from build123d import *

# Parameters (mm, degrees)
F0_W     = 368.677914
F0_H     = 204.665296
F1_DEPTH = 12.7
F2_W     = 368.677914
F2_H     = 204.665296
F2_R     = 96.2279
F3_DEPTH = 12.7
F4_DEPTH = 7.62


with BuildPart() as f1:
    # F0 (on Front) → F1 (new body)
    with BuildSketch(Plane.XZ):
        with Locations((0.233635, 0.70091)):
            Rectangle(F0_W, F0_H)
    extrude(amount=F1_DEPTH)

    # F2 (on face) → F3 (cut)
    with BuildSketch(Plane.XZ.offset(12.7)):
        with Locations((0.233635, 0.70091)):
            Rectangle(F2_W, F2_H)
        Circle(F2_R, mode=Mode.SUBTRACT)
    extrude(amount=-F3_DEPTH, mode=Mode.SUBTRACT)

    # F2 (on face) + F0 (on Front) → F4 (cut)
    with BuildSketch(Plane.XZ.offset(12.7)):
        Circle(F2_R)
    with BuildSketch(Plane.XZ):
        with Locations((0.233635, 0.70091)):
            Rectangle(F0_W, F0_H)
    extrude(amount=-F4_DEPTH, mode=Mode.SUBTRACT)


solid = f1.part
The listing builds one solid part. Answer for the finished solid, in the listing's coordinates (mm). Give positions to 0.01 mm unless a question says otherwise; leave off trailing zeros. Write each loop counter-clockwise with the first axis right and the second up, starting at its lowest first coordinate (ties: lowest second). Pieces come first, ordered by that corner, then holes. Notation, with made-up numbers: (16.25, 8) - (35.25, 8) arc R25 ccw to (35.25, 46) - close; hole circle Ø3 at (-39.75, -20.5). An arc over 180 degrees is marked (long way). One line per question, with ' | ' between items. Start each with the question number.
1. Section A-A, the plane y = -0.8 is taken. Determine the outline of the cut face in (x, z), then the cut area to 3 significant figures.
2. Straight lines are drawn through the part: line 1 (X direction, y = -2.15, z = -2.5); line 2 (Z direction, x = -1, y = -2.05); line 3 (Z direction, x = -65, y = -3.65). For each, find the intervals that lie inside material, in ascending order.
3. Given P1, Ø3, axis at y = -4, z = -62.5, coming from the -X side; P2, Ø1, axis at y = -1.5, z = -73.5, coming from the -X side, each flat-ended and moving along its own axis, determine where each tip first touches the part or whether it passes through.
4. Section C-C, the plane z = 57.5 is taken. Determine the outline of the cut face in (x, y), then the cut area to 3 significant figures.
5. Section B-B, the plane x = 33 is taken. Determine the outline of the cut face in (y, z), then the cut area to 3 significant figures.
Result:
1) outline: circle Ø192.46 at (0, 0) | area: 29,100 mm2
2) line 1: x = -96.2 to 96.2 | line 2: z = -96.22 to 96.22 | line 3: z = -70.96 to 70.96
3) P1: stops at x = -74.42 | P2: stops at x = -62.7
4) outline: (-77.16, -5.08) - (77.16, -5.08) - (77.16, 0) - (-77.16, 0) - close | area: 784 mm2
5) outline: (-5.08, -90.39) - (0, -90.39) - (0, 90.39) - (-5.08, 90.39) - close | area: 918 mm2
